Autodesk Inventor part; units mm, degrees
ref_plane "Arbeitsebene1" through (0, 0, 10) normal (0, 0, 1) x (1, 0, 0)
ref_plane "Arbeitsebene3" through (0, 0, 50) normal (0, 0, 1) x (1, 0, 0)
ref_plane "Arbeitsebene4" through (0, 0, 130) normal (0, 0, 1) x (1, 0, 0)
sketch "Skizze1" plane through (0, 0, 0) normal (0, 0, 1) x (1, 0, 0)
  circle A0 centre (0, 0) radius 30
  circle A1 centre (0, 0) radius 13.5
  circle A2 centre (0, 0) radius 9.5
  circle A3 centre (0, 0) radius 23.25 construction
  line L0 (0, 0) -> (16.4402, 16.4402) construction
  line L1 (0, 0) -> (0, 30) construction
  point P0 (-16.4402, 16.4402)
  point P1 (-16.4402, -16.4402)
  point P2 (16.4402, -16.4402)
  dimension "d3" = 30
  dimension "d4" = 46.5
  dimension "d0" = 4
  dimension "d1" = 27
  dimension "d7" = 360
  dimension "d99" = 45
extrude "Extrusion1" add sketch "Skizze1" along normal blind 15 contours A0 | A1
extrude "Extrusion2" add sketch "Skizze1" against normal blind 2.6 contours A1
sketch "Skizze2" plane through (0, 0, 15) normal (0, 0, 1) x (1, 0, 0)
  point P0 (0, 0)
  point P1 (16.4402, 16.4402)
  point P2 (16.4402, -16.4402)
  point P3 (-16.4402, -16.4402)
  point P4 (-16.4402, 16.4402)
hole "Bohrung1" at (16.4402, 16.4402, 15) at (16.4402, -16.4402, 15) at (-16.4402, -16.4402, 15) at (-16.4402, 16.4402, 15) direction (0, 0, -1) diameter 4.134 end through all
ref_plane "Arbeitsebene1" through (0, 0, 10) normal (0, 0, 1) x (1, 0, 0)
sketch "Skizze10" plane through (0, 0, 15) normal (0, 0, 1) x (1, 0, 0)
  line L0 (-30, 8) -> (30, 8)
  line L1 (30, 8) -> (30, -8)
  line L2 (30, -8) -> (-30, -8)
  line L3 (-30, -8) -> (-30, 8)
  line L4 (-30, 8) -> (30, -8) construction
  line L5 (30, 8) -> (-30, -8) construction
  circle A0 centre (0, 0) radius 30
  circle A1 centre (-16.4402, 16.4402) radius 2.067 construction
  circle A2 centre (-16.4402, -16.4402) radius 2.067 construction
  line L6 (-20, 0) -> (20, 0) construction
  circle A3 centre (0, 0) radius 30
  line L7 (0, 42) -> (0, -42) construction
  point P0 (-28.9137, 8)
  point P1 (-28.9137, -8)
  point P2 (28.9137, -8)
  point P3 (28.9137, 8)
  point P4 (30, 0)
  point P5 (-30, 0)
  dimension "d81" = 16
  dimension "d82" = 40
extrude "Extrusion7" cut sketch "Skizze10" against normal blind 5 contours L0 A0 L3 | L0 A0 L2 | A0 L2 L3 | L0 L1 A0 | L1 L2 A0
sketch "Skizze11" plane through (0, 0, 0) normal (0, 0, -1) x (-1, 0, 0)
  point P0 (0, 0)
  point P1 (-20, 0)
  point P2 (20, 0)
hole "Bohrung4" at (20, 0, 0) at (-20, 0, 0) direction (0, 0, 1) diameter 4.5 end through all countersink diameter 9.4 countersink angle 90
sketch "Skizze4" plane through (0, 0, 0) normal (1, 0, 0) x (0, 1, 0)
  line L0 (9.5, -2.6) -> (-9.5, -2.6) construction
  line L1 (0, 192.52) -> (0, -35.12) construction
  line L2 (-9.5, 15) -> (-9.5, -2.6) construction
  line L3 (9.5, 15) -> (9.5, -2.6) construction
  line L4 (-9.5, 15) -> (9.5, 15) construction
  line L5 (-9.5, 2.4) -> (9.5, 2.4)
  line L6 (-9.5, 2.4) -> (-9.5, 15)
  line L7 (-9.5, 15) -> (-20, 15)
  line L8 (-20, 15) -> (-20, 165)
  line L9 (-20, 165) -> (20, 165)
  line L10 (20, 15) -> (9.5, 15)
  line L11 (9.5, 15) -> (9.5, 2.4)
  line L12 (20, 165) -> (20, 15)
  line L13 (0, 2.4) -> (0, 165)
  point P0 (0, 0)
  dimension "d27" = 5
  dimension "d31" = 150
  dimension "d33" = 40
  dimension "MainAxis_Schluesselweite" = 24
  dimension "d46" = 1
  dimension "d52" = 32
  dimension "Flansch_ParralelMech_FlatPart_Width" = 140
sketch "Skizze7" plane through (0, 0, 50) normal (0, 0, 1) x (1, 0, 0)
  line L0 (-12, 16) -> (-12, -16) construction
  line L1 (-12, 15) -> (-3, 15)
  line L2 (-3, 15) -> (-3, 11.425)
  line L3 (-3, 11.425) -> (3, 11.425)
  line L4 (3, 11.425) -> (3, 15)
  line L5 (3, 15) -> (12, 15)
  line L6 (-12, 0) -> (-12, 15)
  line L7 (0, -16) -> (0, 16) construction
  line L8 (12, -16) -> (12, 16) construction
  line L9 (12, 15) -> (12, 0)
  line L10 (-12, 0) -> (12, 0)
  line L11 (-42, 0) -> (42, 0) construction
  point P0 (0, 11.425)
  point P1 (-12, -7.2111)
  point P2 (12, 7.2111)
  dimension "d51" = 9
  dimension "d63" = 30
  dimension "d64" = 22.85
sketch "Skizze8" plane through (12, -16, 160) normal (1, 0, 0) x (0, 0, -1)
  line L0 (30, -26) -> (30, 58) construction
  line L1 (-32.52, 16) -> (195.12, 16) construction
  point P0 (160, 16)
  point P1 (30, 16)
equation "\"d3\" = Flansch_FemalePart_OuterDia"
equation "\"d4\" = Flansch_FemalePart_HoleDia"
equation "\"d1\" = Flansch_Klemmdeckelausnahme_Dia"
equation "\"d33\" = d28"
equation "\"Total_Bearing_Hole_Dist\" = 80"
properties part number "Flansch_FemalePart_MainAxis_HeadConnectorBase_V2" material "Edelstahl"
The listing builds one solid part. Answer for the finished solid, in the listing's coordinates (mm). A direction names the side the tool comes from. Round coordinates to 2 decimals unless told otherwise and drop trailing zeros. Write each loop counter-clockwise with the first axis right and the second up, starting at its lowest first coordinate (ties: lowest second). Pieces come first, ordered by that corner, then holes. Notation, with made-up numbers: (-3, -23.75) -> (40, -23.75) arc R8 cw to (40, -14.75) -> close; hole circle Ø4 at (-19.75, 82.5). An arc over 180 degrees is marked (long way). Write item = value, one per line.
1) Section D-D on z = 8.5 is taken. Write down the section's boundary in (x, y).
Check values:
outline = circle Ø60 at (0, 0); hole circle Ø4.5 at (-20, 0); hole circle Ø4.13 at (-16.44, -16.44); hole circle Ø4.13 at (-16.44, 16.44); hole circle Ø19 at (0, 0); hole circle Ø4.13 at (16.44, -16.44); hole circle Ø4.13 at (16.44, 16.44); hole circle Ø4.5 at (20, 0)
2) Straight lines are drawn through the part: line 1 along X through (y, z) = (17, 5.5); line 2 along Z through (x, y) = (-7, 15.5); line 3 along Y through (x, z) = (8, 2.25). For each, find the intervals that lie inside material, in ascending order. Write a range as [from, to].
Check values:
line_1 = [-24.72, -18.43], [-14.45, 14.45], [18.43, 24.72]
line_2 = [0, 15]
line_3 = [-28.91, -5.12], [5.12, 28.91]
3) Section C-C on x = -20 is taken. Write down the section's boundary in (y, z), plus the area to 3 significant figures.
Check values:
outline = (-22.36, 0) -> (-4.7, 0) -> (-2.25, 2.45) -> (-2.25, 10) -> (-8, 10) -> (-8, 15) -> (-22.36, 15) -> close; (2.25, 2.45) -> (4.7, 0) -> (22.36, 0) -> (22.36, 15) -> (8, 15) -> (8, 10) -> (2.25, 10) -> close
area = 540 mm²
4) Given pin 1 (5 mm diameter, centred on x = -12.5, y = 2, fed in from +Z); pin 2 (5.5 mm diameter, centred on x = -16.44, y = 16.44, fed in from -Z); pin 3 (2 mm diameter, centred on y = -23, z = 0.5, fed in from -X), each flat-ended and moving along its own axis, determine where each tip first touches the part or whether it passes through.
Check values:
pin_1 = 10
pin_2 = 0
pin_3 = -20.4
5) Which of the six approach directions +Z, -Z, +X, -X, +Y, -Y give full straight-line access (tool end or side, diameter ignored) to faces 1 (the cylindrical face through (-14.6, 15.5, 7.4)), 2 (the flat face through (-18, 2, 10)), 3 (the cylindrical face through (-2.93, -13.18, -1.28))?
Check values:
face_1 = +Z, -Z
face_2 = +Z, +X, -X
face_3 = -Z
6) Section B-B on z = 13.25 is taken. Write down the section's boundary in (x, y), plus the area to 3 significant figures.
Check values:
outline = (-28.91, -8) arc R30 ccw to (28.91, -8) -> (5.12, -8) arc R9.5 cw to (-5.12, -8) -> close; (-28.91, 8) -> (-5.12, 8) arc R9.5 cw to (5.12, 8) -> (28.91, 8) arc R30 ccw to start; hole circle Ø4.13 at (-16.44, -16.44); hole circle Ø4.13 at (-16.44, 16.44); hole circle Ø4.13 at (16.44, -16.44); hole circle Ø4.13 at (16.44, 16.44)
area = 1,800 mm²
7) For a pull along Y with two mould halves and no side action, classify faces 4 (the cylindrical face through (27.712, 11.49, 7.395)), 5 (the flat face through (0, -16, 15)), 6 (the flat face through (17, 0, 10)), 7 (the cylindrical face through (9.061, 2.854, 4.368)) as released by +Y, released by -Y, zero draft, split by the parting line, or undercut.
Check values:
face_4 = split by the parting line
face_5 = zero draft
face_6 = undercut
face_7 = undercut
8) Section A-A on y = 0 is taken. Write down the section's boundary in (x, z), plus the area to 3 significant figures.
Check values:
outline = (-30, 0) -> (-24.7, 0) -> (-22.25, 2.45) -> (-22.25, 10) -> (-30, 10) -> close; (-17.75, 2.45) -> (-15.3, 0) -> (-13.5, 0) -> (-13.5, -2.6) -> (-9.5, -2.6) -> (-9.5, 10) -> (-17.75, 10) -> close; (9.5, -2.6) -> (13.5, -2.6) -> (13.5, 0) -> (15.3, 0) -> (17.75, 2.45) -> (17.75, 10) -> (9.5, 10) -> close; (22.25, 2.45) -> (24.7, 0) -> (30, 0) -> (30, 10) -> (22.25, 10) -> close
area = 329 mm²
